from build123d import *

# Parameters (mm, degrees)
SKETCH1_R                       = 15.175
SKETCH1_R_2                     = 12
SKETCH3_R                       = 12
BOSS_EXTRUDE1_DEPTH             = 2
SKETCH4_R                       = 12
SKETCH4_R_2                     = 9.75
BOSS_EXTRUDE4_DEPTH             = 5
SKETCH6_R                       = 12
SKETCH6_R_2                     = 10.5
BOSS_EXTRUDE5_DEPTH             = 8
SKETCH7_R                       = 2.5
CUT_EXTRUDE2_DEPTH              = 16.1750001
CUT_EXTRUDE2_DEPTH_BACK         = 16.1750001
TAP_DRILL_FOR_M2X0_4_TAP1_D     = 1.6
TAP_DRILL_FOR_M2X0_4_TAP1_DEPTH = 10
TAP_DRILL_FOR_M2X0_4_TAP1_TIP   = 0.480688495


with BuildPart() as part:
    # Sweep1: sweep along a path in Sketch2
    with BuildLine(Plane.XY) as sweep1_path:
        Line((0, 0), (0, -40))
        ThreePointArc((0, -40), (5.857864376, -54.142135624), (20, -60))
        Line((20, -60), (35, -60))
    # Sketch1 → Sweep1 (sweep)
    with BuildSketch(Plane(origin=(0, 0, 0), x_dir=(1, 0, 0), z_dir=(0, 1, 0))):
        Circle(SKETCH1_R)
        Circle(SKETCH1_R_2, mode=Mode.SUBTRACT)
    sweep(path=sweep1_path.line)

    # Sketch3 → Boss-Extrude1 (add)
    with BuildSketch(Plane(origin=(20, 0, 0), x_dir=(0, 0, -1), z_dir=(1, 0, 0))):
        with Locations((0, -60)):
            Circle(SKETCH3_R)
    extrude(amount=BOSS_EXTRUDE1_DEPTH)

    # Sketch4 → Boss-Extrude4 (add)
    with BuildSketch(Plane(origin=(22, 0, 0), x_dir=(0, 0, -1), z_dir=(1, 0, 0))):
        with Locations((0, -60)):
            Circle(SKETCH4_R)
        with Locations((0, -60)):
            Circle(SKETCH4_R_2, mode=Mode.SUBTRACT)
    extrude(amount=BOSS_EXTRUDE4_DEPTH)

    # Sketch6 → Boss-Extrude5 (add)
    with BuildSketch(Plane(origin=(27, 0, 0), x_dir=(0, 0, -1), z_dir=(1, 0, 0))):
        with Locations((0, -60)):
            Circle(SKETCH6_R)
        with Locations((0, -60)):
            Circle(SKETCH6_R_2, mode=Mode.SUBTRACT)
    extrude(amount=BOSS_EXTRUDE5_DEPTH)

    # Sketch7 → Cut-Extrude2 (cut, two sides)
    with BuildSketch(Plane.XY) as cut_extrude2_sk:
        with Locations((0, -20)):
            Circle(SKETCH7_R)
    extrude(amount=CUT_EXTRUDE2_DEPTH, mode=Mode.SUBTRACT)
    extrude(cut_extrude2_sk.sketch, amount=-CUT_EXTRUDE2_DEPTH_BACK, mode=Mode.SUBTRACT)

    # Tap Drill for M2x0.4 Tap1
    with Locations(Plane(origin=(35, 0, 0), x_dir=(0, 0, -1), z_dir=(1, 0, 0))):
        with Locations((0, -47.1625), (12.8375, -60), (0, -72.8375), (-12.8375, -60)):
            Hole(TAP_DRILL_FOR_M2X0_4_TAP1_D / 2, depth=TAP_DRILL_FOR_M2X0_4_TAP1_DEPTH)
            with Locations((0, 0, -(TAP_DRILL_FOR_M2X0_4_TAP1_DEPTH + TAP_DRILL_FOR_M2X0_4_TAP1_TIP / 2))):  # 118° drill point
                Cone(0, TAP_DRILL_FOR_M2X0_4_TAP1_D / 2, TAP_DRILL_FOR_M2X0_4_TAP1_TIP, mode=Mode.SUBTRACT)


solid = part.part
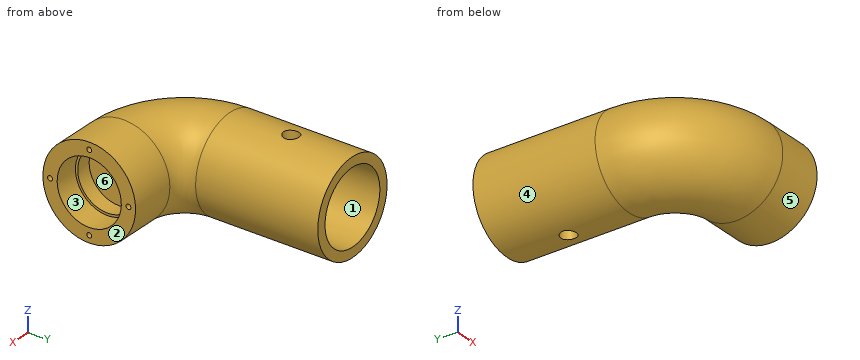
Check sheet for the modelled part. Datum: model origin and axes. Units: mm. Face numbers are marked on the shaded views. A direction names the side the tool comes from. Give positions to 0.01 mm unless a question says otherwise; leave off trailing zeros. Write each loop counter-clockwise with the first axis right and the second up, starting at its lowest first coordinate (ties: lowest second). Pieces come first, ordered by that corner, then holes. Notation, with made-up numbers: (1.5, -28) -> (7.5, -28) arc R23 cw to (7.5, -13) -> close; hole circle Ø4 at (84, -39). An arc over 180 degrees is marked (long way). One line per item, written item: value. Start each with the question number.
Item 1: Draft check along Y on the marked faces 3, 4, 5 and 6. Enter one of: +Y half, -Y half, draft (parallel to the pull), parting line (faces both ways), or undercut.
Item 2: Section check B-B on z = 6. Record the cut outline in (x, y), then the cut area to 3 significant figures.
Item 3: Section check A-A on y = -25. Record the cut outline in (x, z) (3 decimals).
Item 4: Tool access check on the marked faces 1 and 2. Record the directions out of +Z, -Z, +X, -X, +Y, -Y that give a thin tool (end or side, any length) a straight path to the whole face; none if there is none.
Item 5: Gauge pin test, flat ends, axial feed: pin 1 (6 mm diameter, centred on x = -2, y = -60, fed in from +Z); pin 2 (2 mm diameter, centred on y = -62, z = -9.5, fed in from -X); pin 3 (1.4 mm diameter, centred on y = -60, z = -12.84, fed in from -X). Record the tip position at first contact, or that the pin passes through.
Item 6: Section check C-C on x = 0. State how many separate pieces and enclosed holes the cut face has, then the cut area to 3 significant figures.
Item 7: Material ranges on probe 1 along Z at (x, y) = (0.5, -36); probe 2 along Y at (x, z) = (19.5, -4); probe 3 along X at (y, z) = (-23, -8), recorded low to high. Write a range as from..to.
Item 8: Section check D-D on z = -3. Record the cut outline in (x, y), then the cut area to 3 significant figures.
Results list:
1. face 3: undercut
1. face 4: draft
1. face 5: parting line
1. face 6: undercut
2. outline: (-13.94, -40) arc R33.94 ccw to (20, -73.94) -> (35, -73.94) -> (35, -68.62) -> (27, -68.62) -> (27, -67.69) -> (22, -67.69) -> (22, -52.31) -> (27, -52.31) -> (27, -51.38) -> (35, -51.38) -> (35, -46.06) -> (20, -46.06) arc R6.06 cw to (13.94, -40) -> (13.94, 0) -> (10.39, 0) -> (10.39, -40) arc R9.61 ccw to (20, -49.61) -> (20, -70.39) arc R30.39 cw to (-10.39, -40) -> (-10.39, 0) -> (-13.94, 0) -> close
2. area: 710 mm²
3. outline: circle Ø30.35 at (0, 0); hole circle Ø24 at (0, 0)
4. face 1: +Y
4. face 2: +Z, -Z, +X, +Y, -Y
5. pin 1: z = 13.6
5. pin 2: x = -4.38
5. pin 3: x = -1.3
6. separate pieces: 3
6. enclosed holes: 0
6. area: 458 mm²
7. probe 1: -15.17..-11.99, 11.99..15.17
7. probe 2: -74.63..-71.31, -48.67..-45.34
7. probe 3: -12.89..-8.94, 8.94..12.89
8. outline: (-14.88, -40) arc R34.88 ccw to (20, -74.88) -> (35, -74.88) -> (35, -70.06) -> (27, -70.06) -> (27, -69.28) -> (22, -69.28) -> (22, -50.72) -> (27, -50.72) -> (27, -49.94) -> (35, -49.94) -> (35, -45.12) -> (20, -45.12) arc R5.12 cw to (14.88, -40) -> (14.88, 0) -> (11.62, 0) -> (11.62, -40) arc R8.38 ccw to (20, -48.38) -> (20, -71.62) arc R31.62 cw to (-11.62, -40) -> (-11.62, 0) -> (-14.88, 0) -> close
8. area: 658 mm²
